from build123d import *

# Parameters (mm, degrees)
SKETCH1_R               = 150
BOSS_EXTRUDE1_DEPTH     = 500
SKETCH2_R               = 150
SKETCH2_R_2             = 90
CUT_EXTRUDE1_DEPTH      = 70
SKETCH3_W               = 102.450978838
SKETCH3_H               = 18.366336908
CUT_EXTRUDE2_DEPTH      = 151
CUT_EXTRUDE2_DEPTH_BACK = 151
FILLET1_R               = 100
SKETCH4_R               = 67.5
CUT_EXTRUDE3_DEPTH      = 151


with BuildPart() as part:
    # Sketch1 → Boss-Extrude1 (new body)
    with BuildSketch(Plane(origin=(0, 0, 0), x_dir=(1, 0, 0), z_dir=(0, 1, 0))):
        Circle(SKETCH1_R)
    extrude(amount=BOSS_EXTRUDE1_DEPTH)

    # Sketch2 → Cut-Extrude1 (cut)
    with BuildSketch(Plane.XZ):
        Circle(SKETCH2_R)
        Circle(SKETCH2_R_2, mode=Mode.SUBTRACT)
    extrude(amount=-CUT_EXTRUDE1_DEPTH, mode=Mode.SUBTRACT)

    # Sketch3 → Cut-Extrude2 (cut, two sides)
    with BuildSketch(Plane(origin=(0, 0, 0), x_dir=(0, 0, -1), z_dir=(1, 0, 0))) as cut_extrude2_sk:
        with Locations((0, 35)):
            Rectangle(SKETCH3_W, SKETCH3_H)
    extrude(amount=CUT_EXTRUDE2_DEPTH, mode=Mode.SUBTRACT)
    extrude(cut_extrude2_sk.sketch, amount=-CUT_EXTRUDE2_DEPTH_BACK, mode=Mode.SUBTRACT)

    # Fillet1
    fillet1_edges = [part.edges().sort_by_distance(p)[0] for p in [
        (-150, 500, 0),
    ]]
    fillet(fillet1_edges, radius=FILLET1_R)

    # Sketch4 → Cut-Extrude3 (cut, through all)
    with BuildSketch(Plane.XY):
        with Locations((0, 249.430268714)):
            Circle(SKETCH4_R)
    extrude(amount=-CUT_EXTRUDE3_DEPTH, mode=Mode.SUBTRACT)


solid = part.part
Can you work these out from the model? Positions are in its coordinate system, mm. A direction names the side the tool comes from. Give positions to 0.01 mm unless a question says otherwise; leave off trailing zeros. Order: outer loops, then holes, each group sorted by start corner. A loop starts at its lowest first (then second) coordinate and runs counter-clockwise, first axis right, second up. Notation, with made-up numbers: M 48,42 L 52,42 A23 ccw 52,76 Z; hole C -0.5,35 d6. An arc over 180 degrees is marked long. Use a Markdown table: item, result. Add a question column.
Item 1: Will these pins go through, and if not, where does the flat tip stop? pin 1 (4 mm diameter, centred on y = 328.5, z = -32.5, fed in from -X); pin 2 (2 mm diameter, centred on y = 208, z = 116, fed in from +X); pin 3 (10 mm diameter, centred on y = 359, z = -103.5, fed in from -X).
Item 2: If I drill on L1, parallel to Y at x = 0, z = -36.5; L2, parallel to Y at x = 0, z = -105; L3, parallel to X at y = 275, z = -92.5, over which ranges is the centre line in solid material (lowest first)? Write a range as [from, to].
Item 3: Suppose I cut it at C-C (y = 299). List the corners of the cut face in (x, z) for me.
Item 4: Suppose I cut it at A-A (z = -25.5). Count the separate pieces of the cut face and the enclosed holes in it, then the cut area to 3 significant figures.
Item 5: We'd pull the mould along Z, two halves only. Please class faces 4 (the flat face through (65, 70, -65)), 5 (the flat face through (-1, 25.817, 1)), 6 (the flat face through (-1, 250, 0)): +Z half, -Z half, draft (parallel to the pull), parting line (faces both ways), or undercut.
Item 6: For faces 1 (the flat face through (-1, 35, -51.225)), 2 (the cylindrical face through (-71.421, 34.51, -54.764)), 3 (the cylindrical face through (-8.787, 316.356, -73.95)), which set-ups out of +Z, -Z, +X, -X, +Y, -Y let a thin tool reach every point of the face, with its end or its side?
Item 7: Suppose I cut it at B-B (y = 382.5). List the corners of the cut face in (x, z) for me.
Answer sheet:
| question | item | result |
|---|---|---|
| 1 | pin 1 | stops at x = -146.87 |
| 1 | pin 2 | stops at x = 96.31 |
| 1 | pin 3 | stops at x = -113.13 |
| 2 | L1 | y = [0, 25.82], [44.18, 181.93], [316.93, 500] |
| 2 | L2 | y = [70, 181.93], [316.93, 483.52] |
| 2 | L3 | x = [-118.08, -62.47], [62.47, 118.08] |
| 3 | outline | M -45.82,-142.83 L -45.82,0 L 45.82,0 L 45.82,-142.83 A150 ccw long Z |
| 4 | separate pieces | 2 |
| 4 | enclosed holes | 1 |
| 4 | area | 117,000 mm² |
| 5 | face 4 | draft |
| 5 | face 5 | undercut |
| 5 | face 6 | -Z half |
| 6 | face 1 | +X, -X |
| 6 | face 2 | -Y |
| 6 | face 3 | -Z |
| 7 | outline | C 0,0 d300 |
